```python
from build123d import *

# Parameters (mm, degrees)
F0_W     = 500
F0_H     = 500
F1_DEPTH = 3
F3_D     = 10
F5_D     = 12
F7_D     = 12


with BuildPart() as f1:
    # F0 (on Front) → F1 (new body)
    with BuildSketch(Plane.XZ):
        with Locations((250, 250)):
            Rectangle(F0_W, F0_H)
    extrude(amount=F1_DEPTH)

    # F3 (through all)
    with Locations(Plane.XZ.offset(3)):
        with Locations((150, 350), (250, 391.421356), (350, 350), (391.421356, 250), (350, 150), (250, 108.578644), (150, 150), (108.578644, 250)):
            Hole(F3_D / 2)

    # F5 (through all)
    with Locations(Plane.XZ.offset(3)):
        with Locations((25, 325), (25, 475), (175, 475), (325, 475), (475, 475), (475, 325), (475, 175), (475, 25), (325, 25), (175, 25), (25, 25), (25, 175)):
            Hole(F5_D / 2)

    # F7 (through all)
    with Locations(Plane.XZ.offset(3)):
        with Locations((124, 376), (376, 376), (376, 124), (124, 124)):
            Hole(F7_D / 2)


solid = f1.part
```
Geometry check sheet. Reference: the model listing, model coordinates, mm. Coordinates: 2 decimals unless noted, no trailing zeros. Loops run counter-clockwise (first coordinate to the right, second up) from the corner with the lowest first, then second, coordinate; pieces in that order, holes last. Notation, with made-up numbers: (53, -38) -> (72, -38) arc R19 ccw to (72, -25) -> close; hole circle Ø6 at (67.5, -17). An arc over 180 degrees is marked (long way). Put each result on its own line as item: value.
1) Cross-section at B-B on z = 175. Record the boundary of the cut face in (x, y), plus the area to 3 significant figures.
Result set:
outline: (0, -3) -> (19, -3) -> (19, 0) -> (0, 0) -> close; (31, -3) -> (469, -3) -> (469, 0) -> (31, 0) -> close; (481, -3) -> (500, -3) -> (500, 0) -> (481, 0) -> close
area: 1,430 mm^2
2) Cross-section at C-C on x = 25. Record the boundary of the cut face in (y, z).
Result set:
outline: (-3, 0) -> (0, 0) -> (0, 19) -> (-3, 19) -> close; (-3, 31) -> (0, 31) -> (0, 169) -> (-3, 169) -> close; (-3, 181) -> (0, 181) -> (0, 319) -> (-3, 319) -> close; (-3, 331) -> (0, 331) -> (0, 469) -> (-3, 469) -> close; (-3, 481) -> (0, 481) -> (0, 500) -> (-3, 500) -> close
3) Thickness scan on line 1 (Z direction, x = 376, y = -1.65); line 2 (Z direction, x = 475, y = -2.25). Record the ranges inside material, lowest first.
Result set:
line 1: z = 0 to 118, 130 to 370, 382 to 500
line 2: z = 0 to 19, 31 to 169, 181 to 319, 331 to 469, 481 to 500
4) Cross-section at D-D on z = 25. Record the boundary of the cut face in (x, y), plus the area to 3 significant figures.
Result set:
outline: (0, -3) -> (19, -3) -> (19, 0) -> (0, 0) -> close; (31, -3) -> (169, -3) -> (169, 0) -> (31, 0) -> close; (181, -3) -> (319, -3) -> (319, 0) -> (181, 0) -> close; (331, -3) -> (469, -3) -> (469, 0) -> (331, 0) -> close; (481, -3) -> (500, -3) -> (500, 0) -> (481, 0) -> close
area: 1,360 mm^2
5) Cross-section at A-A on x = 325. Record the boundary of the cut face in (y, z), plus the area to 3 significant figures.
Result set:
outline: (-3, 0) -> (0, 0) -> (0, 19) -> (-3, 19) -> close; (-3, 31) -> (0, 31) -> (0, 469) -> (-3, 469) -> close; (-3, 481) -> (0, 481) -> (0, 500) -> (-3, 500) -> close
area: 1,430 mm^2
6) Release check for a two-part mould opening along Z. For faces 1 (the flat face through (247, 0, 254)), 2 (the cylindrical face through (29.76, -1.48, 21.35)), 3 (the cylindrical face through (479.42, -1.48, 329.06)) record: released by +Z, released by -Z, zero draft, split by the parting line, or undercut.
Result set:
face 1: zero draft
face 2: undercut
face 3: undercut
7) Gauge pin test, flat end, axial feed: pin 1 Ø11.5 at (x, z) = (350, 350) entering from +Y. Record the tip position at first contact, or that the pin passes through.
Result set:
pin 1: stops at y = 0
